Verification items for the finished model (mm, model axes). A direction names the side the tool comes from. Round coordinates to 2 decimals unless told otherwise and drop trailing zeros. Loops run counter-clockwise (first coordinate to the right, second up) from the corner with the lowest first, then second, coordinate; pieces in that order, holes last. Notation, with made-up numbers: M 27,-34 L 46,-34 A21 cw 46,-11 Z; hole C 19.5,55 d4. An arc over 180 degrees is marked long. One line per item, written item: value.
from build123d import *

# Parameters (mm, degrees)
SKETCH_1_R          = 11
EXTRUDE_1_DEPTH     = 100
SKETCH_2_R          = 11
SKETCH_2_R_2        = 9
CUT_EXTRUDE_1_DEPTH = 8.5
SKETCH_3_R          = 11
SKETCH_3_R_2        = 10
CUT_EXTRUDE_2_DEPTH = 71.5


with BuildPart() as part:
    # 草圖1 → 填料-伸長1 (new body)
    with BuildSketch(Plane.XY):
        Circle(SKETCH_1_R)
    extrude(amount=EXTRUDE_1_DEPTH)

    # 草圖2 → 除料-伸長1 (cut)
    with BuildSketch(Plane(origin=(0, 0, 0), x_dir=(-1, 0, 0), z_dir=(0, 0, -1))):
        Circle(SKETCH_2_R)
        Circle(SKETCH_2_R_2, mode=Mode.SUBTRACT)
    extrude(amount=-CUT_EXTRUDE_1_DEPTH, mode=Mode.SUBTRACT)

    # 草圖3 → 除料-伸長2 (cut)
    with BuildSketch(Plane.XY.offset(100)):
        Circle(SKETCH_3_R)
        Circle(SKETCH_3_R_2, mode=Mode.SUBTRACT)
    extrude(amount=-CUT_EXTRUDE_2_DEPTH, mode=Mode.SUBTRACT)


solid = part.part
(1) Sectioned sample at A-A on y = 0. Enter the section's corners in (x, z), and give its area (3 significant figures).
Completed:
outline: M -11,8.5 L -9,8.5 L -9,0 L 9,0 L 9,8.5 L 11,8.5 L 11,28.5 L 10,28.5 L 10,100 L -10,100 L -10,28.5 L -11,28.5 Z
area: 2,020 mm^2
(2) Tool access check on faces 1 (the face through (2, -10, 28.5)), 2 (the face through (1.172, 8.923, 4.19)), 3 (the face through (0, 0, 100)). Record the directions out of +Z, -Z, +X, -X, +Y, -Y that give a thin tool (end or side, any length) a straight path to the whole face; none if there is none.
Completed:
face 1: +Z
face 2: -Z
face 3: +Z, +X, -X, +Y, -Y
(3) Thickness scan on L1, parallel to Y at x = -1, z = 15.5; L2, parallel to X at y = 4, z = 14.5; L3, parallel to Y at x = -8, z = 64. Record the ranges inside material, lowest first. Write a range as from..to.
Completed:
L1: y = -10.95..10.95
L2: x = -10.25..10.25
L3: y = -6..6
(4) Depth check by flat-ended pin: pin 1 Ø3 at (x, z) = (-8, 69) entering from -Y; pin 2 Ø5 at (y, z) = (0, 70) entering from -X; pin 3 Ø3 at (y, z) = (-7.5, 81) entering from -X. Enter the tip coordinate at first touch or a pass-through.
Completed:
pin 1: stops at y = -7.6
pin 2: stops at x = -10
pin 3: stops at x = -8
(5) Sectioned sample at C-C on z = 37. Enter the section's corners in (x, y).
Completed:
outline: C 0,0 d20
